Autodesk Inventor part; units mm, degrees
ref_plane "YZ Plane" through (0, 0, 0) normal (1, 0, 0) x (0, 1, 0)
ref_plane "XZ Plane" through (0, 0, 0) normal (0, 1, 0) x (-1, 0, 0)
ref_plane "XY Plane" through (0, 0, 0) normal (0, 0, 1) x (1, 0, 0)
sketch "Sketch1" plane through (0, 0, 0) normal (0, 0, 1) x (1, 0, 0)
  line L0 (-62.5, 37.5) -> (62.5, 37.5)
  line L1 (62.5, 37.5) -> (62.5, -37.5)
  line L2 (62.5, -37.5) -> (-62.5, -37.5)
  line L3 (-62.5, -37.5) -> (-62.5, 37.5)
  point P0 (0, 0)
  point P1 (-62.5, 0)
  point P2 (0, 37.5)
  dimension "d0" = 125
  dimension "d1" = 75
extrude "Extrusion1" add sketch "Sketch1" along normal blind 2
sketch "Sketch2" plane through (0, 0, 2) normal (0, 0, 1) x (1, 0, 0)
  line L0 (-62.5, -37.5) -> (62.5, -37.5)
  line L1 (62.5, -37.5) -> (62.5, 37.5)
  line L2 (62.5, 37.5) -> (-62.5, 37.5)
  line L3 (-62.5, 37.5) -> (-62.5, -37.5)
  line L4 (-59.5, 34.5) -> (59.5, 34.5)
  line L5 (59.5, 34.5) -> (59.5, -34.5)
  line L6 (59.5, -34.5) -> (-59.5, -34.5)
  line L7 (-59.5, -34.5) -> (-59.5, 34.5)
  point P0 (0, 0)
  dimension "d4" = 3
hole "Hole1" at (-59.5, 34.5, 2) at (59.5, 34.5, 2) at (-59.5, -34.5, 2) at (59.5, -34.5, 2) direction (0, 0, -1) diameter 3.4 end through all
fillet "Fillet1" radius 2 4 edges at (-62.5, 37.5, 1) (-62.5, -37.5, 1) (62.5, -37.5, 1) (62.5, 37.5, 1)
sketch "Sketch3" plane through (0, 0, 2) normal (0, 0, 1) x (1, 0, 0)
  line L0 (18.5, 20) -> (45.5, 20)
  line L1 (45.5, 20) -> (45.5, -20)
  line L2 (45.5, -20) -> (18.5, -20)
  line L3 (18.5, -20) -> (18.5, 20)
  line L4 (62.5, -35.5) -> (62.5, 35.5)
  point P0 (0, 0)
  point P1 (18.5, 0)
  dimension "d13" = 27
  dimension "d14" = 40
  dimension "d16" = 17
extrude "Extrusion2" cut sketch "Sketch3" against normal through all
fillet "Fillet2" radius 1.5 4 edges at (18.5, -20, 1) (18.5, 20, 1) (45.5, 20, 1) (45.5, -20, 1)
sketch "Sketch4" plane through (0, 0, 2) normal (0, 0, 1) x (1, 0, 0)
  line L0 (44, 20) -> (20, 20)
  line L1 (44, -20) -> (20, -20)
  line L2 (18.5, -18.5) -> (18.5, 18.5)
  line L3 (20, 20) -> (44, 20)
  line L4 (45.5, 18.5) -> (45.5, -18.5)
  line L5 (14.0041, -17.1435) -> (14.0041, 17.1435)
  line L6 (49.9959, 17.1435) -> (49.9959, -17.1435)
  line L7 (32, 20) -> (32, -20)
  point P0 (0, 0)
  point P1 (14.0041, 0)
  point P2 (49.9959, 0)
  dimension "d21" = 35.9918
hole "Hole2" at (14.0041, 0, 2) at (49.9959, 0, 2) direction (0, 0, -1) diameter 3.4 depth 6 tip angle 118
sketch "Sketch5" plane through (0, 0, 2) normal (0, 0, 1) x (1, 0, 0)
  circle A0 centre (-37.5, 12.5) radius 10.375
  line L0 (-46.325, 17.9553) -> (-46.325, 7.0447)
  line L1 (-62.5, 35.5) -> (-62.5, -35.5)
  line L2 (60.5, 37.5) -> (-60.5, 37.5)
  point P0 (0, 0)
  dimension "d29" = 20.75
  dimension "d30" = 8.825
  dimension "d31" = 25
  dimension "d32" = 25
extrude "Extrusion3" cut sketch "Sketch5" against normal blind 10 contours A0 L0 picked at (-32.9905, 14.9651)
sketch "Sketch6" plane through (0, 0, 2) normal (0, 0, 1) x (1, 0, 0)
  circle A0 centre (-5.5, 12.5) radius 12.75
  line L0 (-16.4, 19.1146) -> (-16.4, 5.8854)
  arc A1 (-46.325, 7.0447) -> (-46.325, 17.9553) centre (-37.5, 12.5) ccw
  point P0 (0, 0)
  dimension "d35" = 25.5
  dimension "d36" = 10.9
  dimension "d37" = 32
extrude "Extrusion4" cut sketch "Sketch6" against normal blind 10 contours A0 L0 picked at (-6.5005, 11.8775)
sketch "Sketch7" plane through (0, 0, 2) normal (0, 0, 1) x (1, 0, 0)
  line L0 (-47.5, -22.5) -> (6.5, -22.5)
  line L1 (-62.5, 35.5) -> (-62.5, -35.5)
  line L2 (-60.5, -37.5) -> (60.5, -37.5)
  line L3 (-34, -12.5) -> (-7, -12.5)
  point P0 (0, 0)
  point P1 (-20.5, -22.5)
  point P2 (-20.5, -12.5)
  dimension "d40" = 54
  dimension "d43" = 15
  dimension "d56" = 15
  dimension "d57" = 10
  dimension "d58" = 27
hole "Hole3" at (-47.5, -22.5, 2) at (6.5, -22.5, 2) at (-20.5, -22.5, 2) at (-34, -12.5, 2) at (-7, -12.5, 2) direction (0, 0, -1) diameter 5.588 end through all
sketch "Sketch8" plane through (0, 0, 0) normal (0, 0, -1) x (-1, 0, 0)
  circle A0 centre (-49.9959, 0) radius 1.7
  circle A1 centre (-14.0041, 0) radius 1.7
  circle A2 centre (-49.9959, 0) radius 3.7
  circle A3 centre (-14.0041, 0) radius 3.7
  point P0 (0, 0)
  dimension "d52" = 2
  dimension "d53" = 2
extrude "Extrusion5" add sketch "Sketch8" along normal blind 5
properties part number "LI0011-IO SHIELD"
The listing builds one solid part. Answer for the finished solid, in the listing's coordinates (mm). A direction names the side the tool comes from. Round coordinates to 2 decimals unless told otherwise and drop trailing zeros. Order: outer loops, then holes, each group sorted by start corner. A loop starts at its lowest first (then second) coordinate and runs counter-clockwise, first axis right, second up. Notation, with made-up numbers: (30.5, 59) -> (68.5, 59) arc R18 cw to (68.5, 66) -> close; hole circle Ø3 at (26.5, 72). An arc over 180 degrees is marked (long way). Put each result on its own line as item: value.
Q1. Each of these flat-tipped pins is pushed along its axis until it touches: P1, Ø7.5, axis at x = -47.5, y = -22.5, coming from the -Z side; P2, Ø2, axis at x = 11.5, z = -2.5, coming from the +Y side. Where does it stop, or does it pass through?
Results list:
P1: z = 0
P2: y = 3.38
Q2. Which of the six approach directions +Z, -Z, +X, -X, +Y, -Y give full straight-line access (tool end or side, diameter ignored) to faces 1 (the cylindrical face through (-60.933, 33.586, 0.986)), 2 (the cylindrical face through (10.475, -1.111, -2.465))?
Results list:
face 1: +Z, -Z
face 2: -Z
Q3. Section A-A, the plane x = 23 is taken. Write down the section's boundary in (y, z).
Results list:
outline: (-37.5, 0) -> (-20, 0) -> (-20, 2) -> (-37.5, 2) -> close; (20, 0) -> (37.5, 0) -> (37.5, 2) -> (20, 2) -> close
Q4. Determine the mould class of faces 3 (the cylindrical face through (57.814, -34.279, 0.986)), 4 (the flat face through (49, -2, -5)) for opening direction X: pulls with the +X half, pulls with the -X half, needs draft (parallel to the pull), parting line crosses it, or undercut.
Results list:
face 3: undercut
face 4: needs draft
Q5. Consider line 1 along Y through (x, z) = (59.5, 1.4); line 2 along X through (y, z) = (-34.5, 0.7); line 3 along X through (y, z) = (-0.5, -0.5). Determine where each line is inside the solid, lowest interval first.
Results list:
line 1: -37.5 to -36.2, -32.8 to 32.8, 36.2 to 37.5
line 2: -62.5 to -61.2, -57.8 to 57.8, 61.2 to 62.5
line 3: 10.34 to 12.38, 15.63 to 17.67, 46.33 to 48.37, 51.62 to 53.66
Q6. Section B-B, the plane y = -12.5 is taken. Write down the section's boundary in (x, z).
Results list:
outline: (-62.5, 0) -> (-36.79, 0) -> (-36.79, 2) -> (-62.5, 2) -> close; (-31.21, 0) -> (-9.79, 0) -> (-9.79, 2) -> (-31.21, 2) -> close; (-4.21, 0) -> (18.5, 0) -> (18.5, 2) -> (-4.21, 2) -> close; (45.5, 0) -> (62.5, 0) -> (62.5, 2) -> (45.5, 2) -> close
Q7. Section C-C, the plane x = -7 is taken. Write down the section's boundary in (y, z), and give its area (3 significant figures).
Results list:
outline: (-37.5, 0) -> (-15.29, 0) -> (-15.29, 2) -> (-37.5, 2) -> close; (-9.71, 0) -> (-0.16, 0) -> (-0.16, 2) -> (-9.71, 2) -> close; (25.16, 0) -> (37.5, 0) -> (37.5, 2) -> (25.16, 2) -> close
area: 88.2 mm^2
Q8. Section D-D, the plane z = -2.5 is taken. Write down the section's boundary in (x, y), and give its area (3 significant figures).
Results list:
outline: circle Ø7.4 at (14, 0); circle Ø7.4 at (50, 0); hole circle Ø3.4 at (14, 0); hole circle Ø3.4 at (50, 0)
area: 67.9 mm^2
